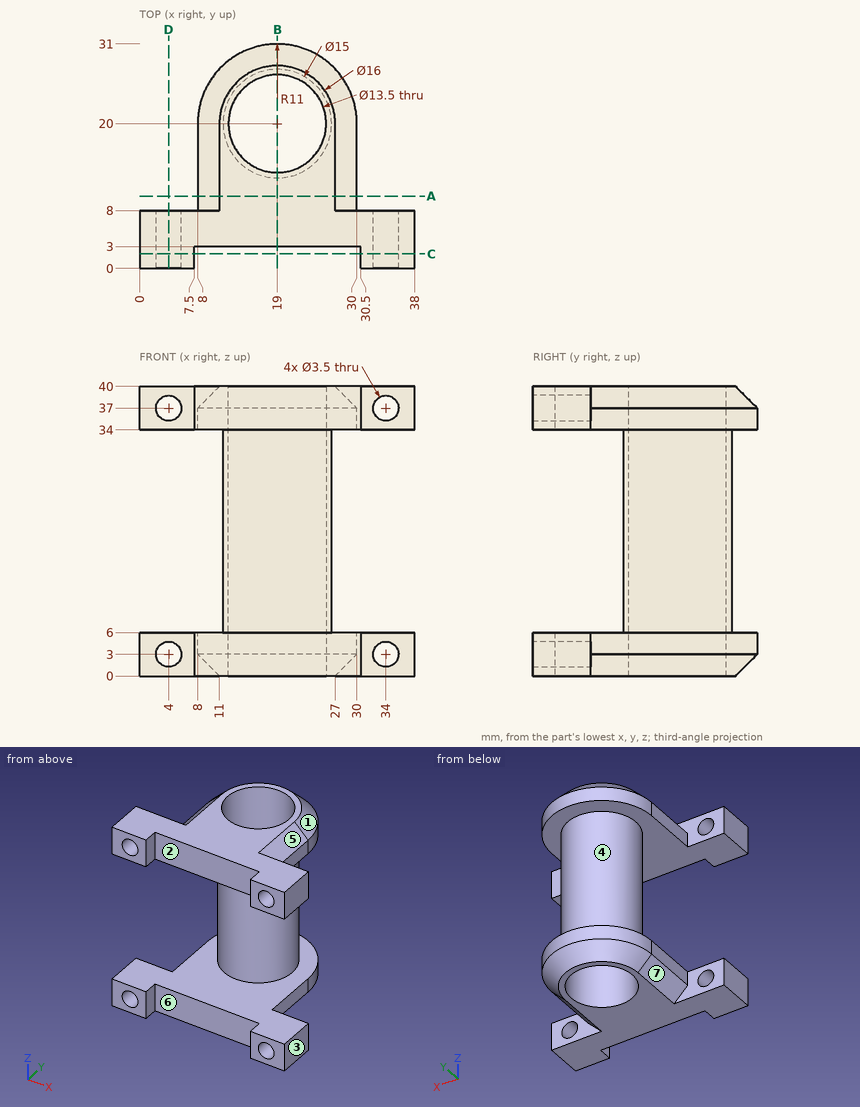
Here's the drawing with two shaded views (mm, measured from the low corner). I have some questions. A direction names the side the tool comes from. Give positions to 0.01 mm unless a question says otherwise; leave off trailing zeros. Loops run counter-clockwise (first coordinate to the right, second up) from the corner with the lowest first, then second, coordinate; pieces in that order, holes last. Notation, with made-up numbers: (52.25, 74.5) - (104.25, 74.5) arc R31 cw to (104.25, 110.5) - close; hole circle Ø6 at (30.25, -20.75). An arc over 180 degrees is marked (long way). Answer in a Markdown table with one row per item. Add a question column.
Q1. If we section it at D-D (x = 4): List the corners of the cut face in (y, z) for me, plus the area to 3 significant figures.
Q2. If we section it at B-B (x = 19): List the corners of the cut face in (y, z) for me, plus the area to 3 significant figures.
Q3. We'd pull the mould along X, two halves only. Please class the marked faces 1, 2 and 3: +X half, -X half, draft (parallel to the pull), parting line (faces both ways), or undercut.
Q4. Which directions (+Z, -Z, +X, -X, +Y, -Y) give clear straight access to the entire face, cutting with the end or side of a thin tool? Please do the marked faces 4, 5, 6 and 7.
Q5. If we section it at A-A (y = 10): List the corners of the cut face in (x, z) for me.
Q6. Please list where these lines run through material, in increasing order: L1, parallel to X at y = 2, z = 3; L2, parallel to Z at x = 21.5, y = 8.5; L3, parallel to X at y = 3.5, z = 37. Write a range as from..to.
Q7. If we section it at C-C (y = 2): List the corners of the cut face in (x, z) for me, plus the area to 3 significant figures.
Q8. For pin 1 (1.8 mm diameter, centred on x = 16, z = 38.5, fed in from -Y); pin 2 (0.9 mm diameter, centred on y = 16.5, z = 5, fed in from -X); pin 3 (6 mm diameter, centred on y = 26, z = 8.5, fed in from -X); pin 4 (2 mm diameter, centred on x = 34, z = 37, fed in from +Y), each with a flat end and sliding along its axis, tell me the tip position at first contact or that it passes through.
The answers:
| question | item | result |
|---|---|---|
| 1 | outline | (0, 0) - (8, 0) - (8, 1.25) - (0, 1.25) - close; (0, 4.75) - (8, 4.75) - (8, 6) - (0, 6) - close; (0, 34) - (8, 34) - (8, 35.25) - (0, 35.25) - close; (0, 38.75) - (8, 38.75) - (8, 40) - (0, 40) - close |
| 1 | area | 40.0 mm^2 |
| 2 | outline | (3, 0) - (13.25, 0) - (13.25, 40) - (3, 40) - (3, 34) - (12.5, 34) - (12.5, 6) - (3, 6) - close; (26.75, 0) - (28, 0) - (31, 3) - (31, 6) - (27.5, 6) - (27.5, 34) - (31, 34) - (31, 37) - (28, 40) - (26.75, 40) - close |
| 2 | area | 207 mm^2 |
| 3 | face 1 | parting line |
| 3 | face 2 | undercut |
| 3 | face 3 | +X half |
| 4 | face 4 | none |
| 4 | face 5 | +Z, +X, +Y |
| 4 | face 6 | +Z, -Z, -Y |
| 4 | face 7 | -Z, -X, +Y |
| 5 | outline | (8, 3) - (11, 0) - (27, 0) - (30, 3) - (30, 6) - (8, 6) - close; (8, 34) - (30, 34) - (30, 37) - (27, 40) - (11, 40) - (8, 37) - close |
| 6 | L1 | x = 0..2.25, 5.75..7.5, 30.5..32.25, 35.75..38 |
| 6 | L2 | z = 0..6, 34..40 |
| 6 | L3 | x = 0..2.25, 5.75..32.25, 35.75..38 |
| 7 | outline | (0, 0) - (7.5, 0) - (7.5, 6) - (0, 6) - close; (0, 34) - (7.5, 34) - (7.5, 40) - (0, 40) - close; (30.5, 0) - (38, 0) - (38, 6) - (30.5, 6) - close; (30.5, 34) - (38, 34) - (38, 40) - (30.5, 40) - close; hole circle Ø3.5 at (4, 3); hole circle Ø3.5 at (4, 37); hole circle Ø3.5 at (34, 3); hole circle Ø3.5 at (34, 37) |
| 7 | area | 142 mm^2 |
| 8 | pin 1 | stops at y = 3 |
| 8 | pin 2 | stops at x = 8 |
| 8 | pin 3 | stops at x = 8.89 |
| 8 | pin 4 | passes through |
